Geometry: final body of the model. Coordinates: model frame, mm. Face numbers are marked on the shaded views. A direction names the side the tool comes from. Coordinates: 2 decimals unless noted, no trailing zeros. Loops run counter-clockwise (first coordinate to the right, second up) from the corner with the lowest first, then second, coordinate; pieces in that order, holes last. Notation, with made-up numbers: (37.25, 12.25) -> (45.25, 12.25) arc R20 ccw to (45.25, 33.25) -> close; hole circle Ø1 at (25.25, 81). An arc over 180 degrees is marked (long way). One line per item, written item: value. Start each with the question number.
Item 1: Section query D-D on x = 37.5. Return loops of the section in (y, z), then the cut area to 3 significant figures.
Item 2: Section query B-B on x = 4.5. Return loops of the section in (y, z).
Item 3: Section query A-A on y = 7. Return loops of the section in (x, z), then the cut area to 3 significant figures.
Item 4: Section query C-C on z = 10. Return loops of the section in (x, y), then the cut area to 3 significant figures.
Item 5: Set-up query: the marked faces 1, 2, 3, 4 and 5. Return all of +Z, -Z, +X, -X, +Y, -Y with unobstructed straight access to the full face (end or side cutting, diameter ignored); none if empty.
Item 6: Contact query for flat-ended pins moving along their axis: pin 1 Ø4 at (x, y) = (4.5, 40) entering from +Z; pin 2 Ø5.5 at (y, z) = (35.5, 11) entering from +X; pin 3 Ø10 at (x, z) = (10.5, 6.5) entering from +Y; pin 4 Ø12 at (x, z) = (7.5, 4.5) entering from +Y. Output: stop coordinate, or through.
Item 7: Mould query, pull axis Z, two halves, no side actions, for the marked faces 6, 7 and 8. Classes: +Z half, -Z half, draft (parallel to the pull), parting line (faces both ways), or undercut.
Item 8: Ray query, probe 1 along Y at (x, z) = (4.5, 18.6); probe 2 along X at (y, z) = (28.5, 7); probe 3 along X at (y, z) = (40, 18.6). Return the intervals inside material, ascending. Write a range as from..to.
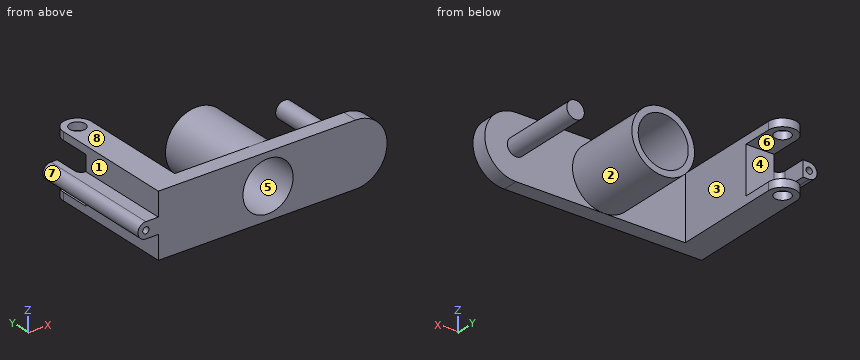
Autodesk Inventor part; units mm, degrees
ref_plane "YZ Plane" through (0, 0, 0) normal (1, 0, 0) x (0, 1, 0)
ref_plane "XZ Plane" through (0, 0, 0) normal (0, 1, 0) x (-1, 0, 0)
ref_plane "XY Plane" through (0, 0, 0) normal (0, 0, 1) x (1, 0, 0)
sketch "Sketch1" plane through (0, 0, 0) normal (0, 0, 1) x (1, 0, 0)
  line L0 (0, 0) -> (0, 40)
  line L1 (0, 0) -> (63, 0)
  line L2 (63, 0) -> (63, 5)
  line L3 (63, 5) -> (9, 5)
  arc A0 (9, 40) -> (0, 40) centre (4.5, 40) ccw
  line L4 (9, 40) -> (9, 5)
  circle A1 centre (4.5, 40) radius 2.5
  dimension "d0" = 40
  dimension "d2" = 5
  dimension "d6" = 4.5
  dimension "d7" = 5
  dimension "d8" = 9
  dimension "d9" = 54
  dimension "d47" = 32.5
extrude "Extrusion1" add sketch "Sketch1" along normal blind 20
sketch "Sketch2" plane through (9, 5, 0) normal (0, 1, 0) x (1, 0, 0)
  line L0 (0, 0) -> (0, -20)
  circle A0 centre (26, -10) radius 10
  line L1 (0, 0) -> (54, 0)
  circle A1 centre (54, -10) radius 2.8
  line L2 (54, 0) -> (54, -20)
  point P0 (-9, 0)
  dimension "d14" = 20
  dimension "d16" = 26
  dimension "d20" = 5.6
  dimension "d21" = 10
  dimension "d22" = 15.2
  dimension "d67" = 0
sketch "Sketch7" plane through (9, 5, 0) normal (1, 0, 0) x (0, 0, -1)
  line L0 (-10, 41.0364) -> (-10, 39.6436)
  line L1 (0, 39.5) -> (-20, 39.5)
  line L2 (-2.5, 39.5) -> (-2.5, 25.5)
  line L3 (-17.5, 39.5) -> (-17.5, 25.5)
  line L4 (-17.5, 39.5) -> (-2.5, 39.5)
  line L5 (0, 32.5) -> (-20, 32.5)
  line L6 (-17.5, 25.5) -> (-2.5, 25.5)
  point P0 (0, -5)
  dimension "d40" = 14
  dimension "d41" = 14
  dimension "d42" = 15
extrude "Extrusion5" cut sketch "Sketch7" against normal blind 14
extrude "Extrusion6" add sketch "Sketch2" along normal blind 25
sketch "Sketch9" plane through (35, 30, 10) normal (0, 1, 0) x (1, 0, 0)
  circle A0 centre (0, 0) radius 8
  point P0 (-35, 10)
  dimension "d50" = 16
extrude "Extrusion7" cut sketch "Sketch9" against normal blind 31
sketch "Sketch12" plane through (35, 5, 0) normal (0, 1, 0) x (1, 0, 0)
  line L0 (28, 0) -> (28, -20)
  arc A0 (28, -20) -> (28, 0) centre (28, -10) ccw
  line L1 (28, 0) -> (-35, 0)
  line L2 (28, 0) -> (28, -20)
extrude "Extrusion10" add sketch "Sketch12" against normal blind 5
sketch "Sketch13" plane through (0, 0, 0) normal (0, -1, 0) x (1, 0, 0)
  circle A0 centre (-4, 10) radius 1
  line L0 (-4, 12.5) -> (0, 12.5)
  line L1 (0, 0) -> (0, 20)
  line L2 (-4, 7.5) -> (0, 7.5)
  arc A1 (-4, 12.5) -> (-4, 7.5) centre (-4, 10) ccw
  line L3 (0, 7.5) -> (0, 12.5)
  line L4 (63, 0) -> (0, 0)
  line L5 (0, 20) -> (63, 20)
  dimension "d68" = 2
  dimension "d72" = 4
  dimension "d73" = 10
  dimension "d74" = 20
extrude "Extrusion11" add sketch "Sketch13" against normal blind 40
sketch "Sketch14" plane through (-4, 0, 12.5) normal (0, 0, 1) x (1, 0, 0)
  line L0 (0, 40) -> (4, 40)
  line L1 (13, 30.5) -> (4, 30.5)
  line L2 (4, 40) -> (4, 30.5)
  line L3 (4, 30.5) -> (2, 30.5)
  line L4 (2, 30.5) -> (2, 40)
  line L5 (2, 40) -> (4, 40)
  point P0 (4, 0)
  dimension "d75" = 2
extrude "Extrusion12" cut sketch "Sketch14" against normal up to surface (5 mm away)
fillet "Fillet4" radius 2 1 edges at (-2, 30.5, 10)
equation "\"d21\" = d19"
equation "\"d40\" = d41"
equation "\"d73\" = 0.5 * d74"
equation "\"d19\" = 0.5 * d14"
properties part number "ValveBaseMk2.5"
Reply:
1. outline: (0, 0) -> (5, 0) -> (5, 0.32) -> (30, 0.32) -> (30, 2.4) -> (0, 2.4) -> close; (0, 17.6) -> (30, 17.6) -> (30, 19.68) -> (5, 19.68) -> (5, 20) -> (0, 20) -> close
1. area: 128 mm²
2. outline: (0, 0) -> (37.5, 0) -> (37.5, 2.5) -> (30.5, 2.5) -> (30.5, 17.5) -> (37.5, 17.5) -> (37.5, 20) -> (0, 20) -> close; (42.5, 0) -> (44.5, 0) -> (44.5, 2.5) -> (42.5, 2.5) -> close; (42.5, 17.5) -> (44.5, 17.5) -> (44.5, 20) -> (42.5, 20) -> close
3. outline: (-4, 7.5) -> (0, 7.5) -> (0, 0) -> (9, 0) -> (9, 20) -> (0, 20) -> (0, 12.5) -> (-4, 12.5) arc R2.5 ccw to start; circle Ø20 at (35, 10); circle Ø5.6 at (63, 10); hole circle Ø2 at (-4, 10); hole circle Ø16 at (35, 10)
3. area: 344 mm²
4. outline: (-6.5, 0) -> (-5, 0) -> (-5, 40) -> (-6.5, 40) -> close; (-3, 0) -> (27, 0) -> (27, 30) -> (25, 30) -> (25, 5) -> (9, 5) -> (9, 30.5) -> (0, 30.5) arc R2 cw to (-2, 32.5) -> (-2, 40) -> (-3, 40) -> close; (43, 0) -> (73, 0) -> (73, 5) -> (65.8, 5) -> (65.8, 30) -> (60.2, 30) -> (60.2, 5) -> (45, 5) -> (45, 30) -> (43, 30) -> close
4. area: 916 mm²
5. face 1: +Z, -X, +Y, -Y
5. face 2: +Y
5. face 3: +Z, -Z, +Y
5. face 4: +X, +Y
5. face 5: +Y, -Y
6. pin 1: passes through
6. pin 2: stops at x = -2
6. pin 3: stops at y = 43.35
6. pin 4: stops at y = 44.5
7. face 6: undercut
7. face 7: parting line
7. face 8: +Z half
8. probe 1: y = 0..37.5, 42.5..44.5
8. probe 2: x = 0..9, 25.46..27.58, 42.42..44.54
8. probe 3: x = 0..2, 7..9
